Can you work these out from the model? Positions are in its coordinate system, mm. Face numbers are marked on the shaded views. A direction names the side the tool comes from. Give positions to 0.01 mm unless a question says otherwise; leave off trailing zeros. Loops run counter-clockwise (first coordinate to the right, second up) from the corner with the lowest first, then second, coordinate; pieces in that order, holes last. Notation, with made-up numbers: M 32.25,43.25 L 89.25,43.25 A23 ccw 89.25,56.25 Z; hole C 17.25,38 d8. An arc over 180 degrees is marked long. Use CSV: the item, a comma, the result in double quotes.
from build123d import *

# Parameters (mm, degrees)
BOSS_EXTRUDE1_DEPTH = 16.51
SKETCH2_R           = 1.651
CUT_EXTRUDE1_DEPTH  = 16.51
SKETCH3_W           = 30.48
SKETCH3_H           = 45.72
CUT_EXTRUDE2_DEPTH  = 13.335


with BuildPart() as part:
    # Sketch1 → Boss-Extrude1 (new body)
    with BuildSketch(Plane(origin=(0, 0, 0), x_dir=(1, 0, 0), z_dir=(0, 1, 0))):
        Polygon((-26.766598834, -7.489394136), (-4.769553578, 30.610605864), (27.43635591, 30.610605864), (49.433401166, -7.489394136), (49.433401166, -15.109394136), (-26.766598834, -15.109394136), align=None)
        Polygon((-17.967780731, -7.489394136), (40.634583064, -7.489394136), (23.036946859, 22.990605864), (-0.370144526, 22.990605864), align=None, mode=Mode.SUBTRACT)
    extrude(amount=BOSS_EXTRUDE1_DEPTH)

    # Sketch2 → Cut-Extrude1 (cut)
    with BuildSketch(Plane(origin=(0, 16.51, 0), x_dir=(1, 0, 0), z_dir=(0, 1, 0))):
        with Locations(Location((-22.702598834, -11.299394136, 0), (0, 0, 270))):
            Circle(SKETCH2_R)
        with Locations(Location((45.369401166, -11.299394136, 0), (0, 0, 270))):
            Circle(SKETCH2_R)
    extrude(amount=-CUT_EXTRUDE1_DEPTH, mode=Mode.SUBTRACT)

    # Sketch3 → Cut-Extrude2 (cut)
    with BuildSketch(Plane(origin=(0, 16.51, 0), x_dir=(1, 0, 0), z_dir=(0, 1, 0))):
        with Locations((11.359446422, 7.750605864)):
            Rectangle(SKETCH3_W, SKETCH3_H)
    extrude(amount=-CUT_EXTRUDE2_DEPTH, mode=Mode.SUBTRACT)


solid = part.part
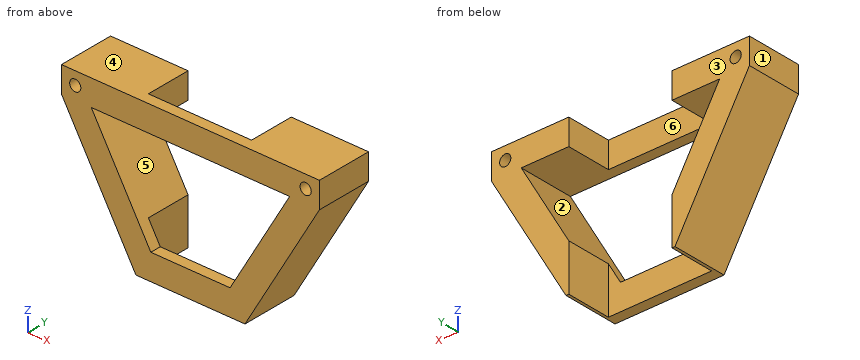
Q1. If we mould it in two halves opening along X, with no side actions, what happens to the marked faces 1, 2 and 3? For each: released by +X, released by -X, zero draft, split by the parting line, or undercut.
Model answer:
face 1,"released by -X"
face 2,"undercut"
face 3,"zero draft"
Q2. I want a section at C-C, the plane z = 11. Please give me the cut outline in (x, y) (3 decimals).
Model answer:
outline,"M -26.767,0 L -24.326,0 L -24.326,16.51 L -26.767,16.51 Z; M -21.079,0 L 43.746,0 L 43.746,16.51 L 26.599,16.51 L 26.599,3.175 L -3.881,3.175 L -3.881,16.51 L -21.079,16.51 Z; M 46.993,0 L 49.433,0 L 49.433,16.51 L 46.993,16.51 Z"
Q3. For the marked faces 4, 5 and 6, which set-ups out of +Z, -Z, +X, -X, +Y, -Y let a thin tool reach every point of the face, with its end or its side?
Model answer:
face 4,"+Z, +X, -X, +Y, -Y"
face 5,"+Y, -Y"
face 6,"+Z, -Z, +Y"
Q4. I want a section at A-A, the plane x = 13.5. Please give me the cut outline in (y, z) (3 decimals).
Model answer:
outline,"M 0,-30.611 L 3.175,-30.611 L 3.175,-22.991 L 0,-22.991 Z; M 0,7.489 L 3.175,7.489 L 3.175,15.109 L 0,15.109 Z"
Q5. Please list where these lines run through material, in increasing order: L1, parallel to X at y = 9.75, z = 13.5; L2, parallel to X at y = 15.5, z = 10; L3, parallel to Z at x = -12.5, y = 1.75. Write a range as from..to.
Model answer:
L1,"-26.77..-3.88, 26.6..49.43"
L2,"-26.77..-23.72, -21.68..-3.88, 26.6..44.35, 46.39..49.43"
L3,"-17.22..-1.98, 7.49..15.11"
Q6. I want a section at B-B, the plane y = 11.5. Please give me the cut outline in (x, z), then the cut area to 3 significant figures.
Model answer:
outline,"M -26.77,7.49 L -4.77,-30.61 L -3.88,-30.61 L -3.88,-16.91 L -17.97,7.49 L -3.88,7.49 L -3.88,15.11 L -26.77,15.11 Z; M 26.6,-30.61 L 27.44,-30.61 L 49.43,7.49 L 49.43,15.11 L 26.6,15.11 L 26.6,7.49 L 40.63,7.49 L 26.6,-16.82 Z; hole C -22.7,11.3 d3.3; hole C 45.37,11.3 d3.3"
area,"893 mm2"
Q7. I'm going to push flat-ended pins straight in: P1, Ø8.5, axis at x = 17, z = 11.5, coming from the +Y side (3 decimals); P2, Ø4, axis at x = -15.5, y = 12, coming from the -Z side; P3, Ø4, axis at y = 9, z = -26, coming from the -X side. Where does each tip first touch, or does it pass through?
Model answer:
P1,"y = 3.175"
P2,"z = -15.49"
P3,"x = -8.59"
Q8. I want a section at D-D, the plane z = -5.5. Please give me the cut outline in (x, y), then the cut area to 3 significant figures.
Model answer:
outline,"M -19.27,0 L -10.47,0 L -10.47,16.51 L -19.27,16.51 Z; M 33.14,0 L 41.93,0 L 41.93,16.51 L 33.14,16.51 Z"
area,"291 mm2"
